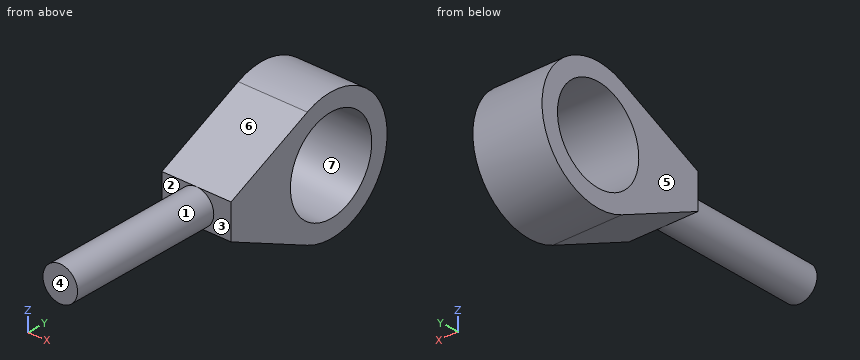
```python
from build123d import *

# Parameters (mm, degrees)
SKETCH2_R                = 4.7625
BOSS_EXTRUDE1_DEPTH      = 42.545
SKETCH3_R                = 12.7
BOSS_EXTRUDE2_DEPTH      = 9.525
BOSS_EXTRUDE2_DEPTH_BACK = 9.525


with BuildPart() as part:
    # Sketch2 → Boss-Extrude1 (new body)
    with BuildSketch(Plane(origin=(0, 0, 0), x_dir=(1, 0, 0), z_dir=(0, 1, 0))):
        Circle(SKETCH2_R)
    extrude(amount=BOSS_EXTRUDE1_DEPTH)

    # Sketch3 → Boss-Extrude2 (add, two sides)
    with BuildSketch(Plane(origin=(0, 0, 0), x_dir=(0, 0, -1), z_dir=(1, 0, 0))) as boss_extrude2_sk:
        with BuildLine():
            Line((-4.7625, 42.545), (-15.875, 66.375833154))
            ThreePointArc((-15.875, 66.375833154), (0, 91.294591691), (15.875, 66.375833154))
            Line((15.875, 66.375833154), (4.7625, 42.545))
            Line((4.7625, 42.545), (-4.7625, 42.545))
        make_face()
        with Locations((0, 73.778467227)):
            Circle(SKETCH3_R, mode=Mode.SUBTRACT)
    extrude(amount=BOSS_EXTRUDE2_DEPTH)
    extrude(boss_extrude2_sk.sketch, amount=-BOSS_EXTRUDE2_DEPTH_BACK)


solid = part.part
```
Part model, mm, in its own coordinate system. Face numbers are marked on the shaded views. A direction names the side the tool comes from. Round coordinates to 2 decimals unless told otherwise and drop trailing zeros. Write each loop counter-clockwise with the first axis right and the second up, starting at its lowest first coordinate (ties: lowest second). Pieces come first, ordered by that corner, then holes.
Item 1: Two-plate mould, pull along Z, no slides. Class the marked faces 5, 6 and 7: +Z half, -Z half, draft (parallel to the pull), parting line (faces both ways), or undercut.
Results:
face 5: draft
face 6: +Z half
face 7: undercut
Item 2: Cut at C-C, the plane y = 72. Give the cut face in (x, z) (3 decimals).
Results:
outline: (-9.525, -17.426) - (9.525, -17.426) - (9.525, -12.575) - (-9.525, -12.575) - close; (-9.525, 12.575) - (9.525, 12.575) - (9.525, 17.426) - (-9.525, 17.426) - close
Item 3: Cut at B-B, the plane x = 2. Give the cut face in (y, z) (1 decimal).
Results:
outline: (0, -4.3) - (42.5, -4.3) - (42.5, -4.8) - (66.4, -15.9) arc R17.5 ccw (long way) to (66.4, 15.9) - (42.5, 4.8) - (42.5, 4.3) - (0, 4.3) - close; hole circle Ø25.4 at (73.8, 0)
Item 4: Probe L1, parallel to Y at x = -3.25, z = 6.5; L2, parallel to Y at x = 0.5, z = -7; L3, parallel to Z at x = 1, y = 41. List the from-to ranges inside material, lowest first.
Results:
L1: y = 46.27 to 62.87, 84.69 to 90.04
L2: y = 47.34 to 63.18, 84.38 to 89.84
L3: z = -4.66 to 4.66
Item 5: Which spindle directions (+Z, -Z, +X, -X, +Y, -Y) get a long thin tool onto all of the face, cutting with end or side? Do the marked faces 1, 2, 3 and 4. Say none if no direction does.
Results:
face 1: -Y
face 2: -X, -Y
face 3: +X, -Y
face 4: +Z, -Z, +X, -X, -Y
Item 6: Drop flat-ended pins along their axis: pin 1 Ø1 at (x, y) = (1, 13.5) entering from +Z; pin 2 Ø4 at (x, z) = (-6, -0.5) entering from +Y; pin 3 Ø5 at (x, y) = (-2.5, 17) entering from +Z; pin 4 Ø3 at (y, z) = (40.5, 3.5) entering from -X. Give the stop position or say it passes through.
Results:
pin 1: stops at z = 4.74
pin 2: stops at y = 91.29
pin 3: stops at z = 4.76
pin 4: stops at x = -4.32
Item 7: Cut at D-D, the plane z = 9. Give the cut face in (x, y) (3 decimals), plus the area to 3 significant figures.
Results:
outline: (-9.525, 51.632) - (9.525, 51.632) - (9.525, 64.818) - (-9.525, 64.818) - close; (-9.525, 82.739) - (9.525, 82.739) - (9.525, 88.806) - (-9.525, 88.806) - close
area: 367 mm2
Item 8: Cut at A-A, the plane z = 0. Give the cut face in (x, y) (1 decimal), plus the area to 3 significant figures.
Results:
outline: (-9.5, 42.5) - (-4.8, 42.5) - (-4.8, 0) - (4.8, 0) - (4.8, 42.5) - (9.5, 42.5) - (9.5, 61.1) - (-9.5, 61.1) - close; (-9.5, 86.5) - (9.5, 86.5) - (9.5, 91.3) - (-9.5, 91.3) - close
area: 850 mm2
